```python
from build123d import *

# Parameters (mm, degrees)
F0_W     = 100
F0_H     = 200
F0_W_2   = 120
F0_H_2   = 21.92845
F1_DEPTH = 10


with BuildPart() as f1:
    # F0 (on Top) → F1 (new body)
    with BuildSketch(Plane.XY):
        Polygon((84.464286, -7.5), (85, -7.5), (85, 7.5), align=None)
        Polygon((60, -692.5), (84.464286, -7.5), (0, -7.5), (0, -154.242083), (-50, -154.242083), (-50, -7.5), (-84.464286, -7.5), (-60, -692.5), (-60, -670.57155), (60, -670.57155), align=None)
        with Locations((0, -538.492203)):
            Rectangle(F0_W, F0_H, mode=Mode.SUBTRACT)
        Polygon((0, -7.5), (84.464286, -7.5), (85, 7.5), (-85, 7.5), (-84.464286, -7.5), (-50, -7.5), (-50, -4.242083), (0, -4.242083), align=None)
        with Locations((0, -681.535775)):
            Rectangle(F0_W_2, F0_H_2)
        Polygon((-84.464286, -7.5), (-85, 7.5), (-85, -7.5), align=None)
    extrude(amount=F1_DEPTH)


solid = f1.part
```
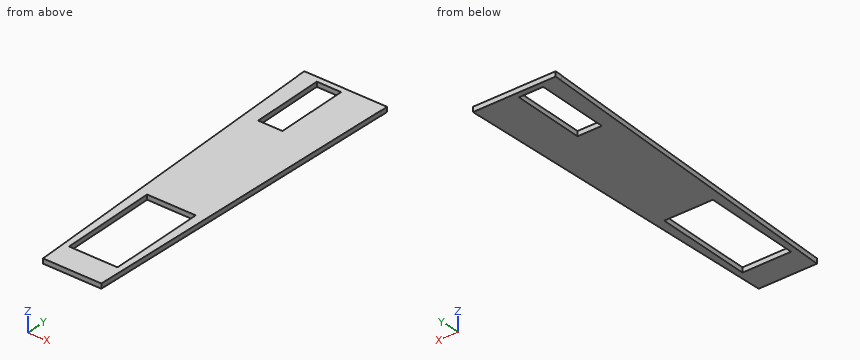
The listing builds one solid part. Answer for the finished solid, in the listing's coordinates (mm). Give positions to 0.01 mm unless a question says otherwise; leave off trailing zeros. Order: outer loops, then holes, each group sorted by start corner. A loop starts at its lowest first (then second) coordinate and runs counter-clockwise, first axis right, second up. Notation, with made-up numbers: (64, 70.25) - (71, 70.25) arc R23 ccw to (71, 96.25) - close; hole circle Ø4 at (15.25, 34). An arc over 180 degrees is marked (long way). Answer in a Markdown table with one row per item. Add a question column.
Q1. The part is cut by section A-A (x = 39). Determine the outline of the cut face in (y, z), then the cut area to 3 significant figures.
Q2. The part is cut by section C-C (y = -458.5). Determine the outline of the cut face in (x, z).
Q3. Find the intervals of material crossed by line 1 along Y through (x, z) = (-36, 5.5); line 2 along Y through (x, z) = (43, 3.75); line 3 along X through (y, z) = (-626, 8) (3 decimals), in increasing order. Write a range as [from, to].
Q4. Given P1, Ø3, axis at y = -562.5, z = 3, coming from the +X side; P2, Ø5, axis at y = -213.5, z = 8.5, coming from the -X side; P3, Ø3, axis at y = -353, z = 6.5, coming from the +X side, each flat-ended and moving along its own axis, determine where each tip first touches the part or whether it passes through.
Q5. The part is cut by section B-B (z = 5.5). Determine the outline of the cut face in (x, y).
Q6. The part is cut by section D-D (y = -202.5). Determine the outline of the cut face in (x, z).
Determined:
| question | item | result |
|---|---|---|
| 1 | outline | (-692.5, 0) - (-638.49, 0) - (-638.49, 10) - (-692.5, 10) - close; (-438.49, 0) - (7.5, 0) - (7.5, 10) - (-438.49, 10) - close |
| 1 | area | 5,000 mm² |
| 2 | outline | (-68.36, 0) - (-50, 0) - (-50, 10) - (-68.36, 10) - close; (50, 0) - (68.36, 0) - (68.36, 10) - (50, 10) - close |
| 3 | line 1 | y = [-692.5, -638.49], [-438.49, -154.24], [-4.24, 7.5] |
| 3 | line 2 | y = [-692.5, -638.49], [-438.49, 7.5] |
| 3 | line 3 | x = [-62.375, -50], [50, 62.375] |
| 4 | P1 | stops at x = 64.7 |
| 4 | P2 | stops at x = -77.2 |
| 4 | P3 | stops at x = 72.18 |
| 5 | outline | (-85, -7.5) - (-84.46, -7.5) - (-60, -692.5) - (60, -692.5) - (84.46, -7.5) - (85, -7.5) - (85, 7.5) - (-85, 7.5) - close; hole (-50, -638.49) - (50, -638.49) - (50, -438.49) - (-50, -438.49) - close; hole (-50, -154.24) - (0, -154.24) - (0, -4.24) - (-50, -4.24) - close |
| 6 | outline | (-77.5, 0) - (77.5, 0) - (77.5, 10) - (-77.5, 10) - close |
